Design review of the part built by this model. Coordinates are the model's own, in mm. A direction names the side the tool comes from. Coordinates: 2 decimals unless noted, no trailing zeros. Loops run counter-clockwise (first coordinate to the right, second up) from the corner with the lowest first, then second, coordinate; pieces in that order, holes last.
Q1. Draft analysis for pull direction Y (two halves, no side actions). For faces 1 (the face through (-9.425, -6.386, 1.479)), 2 (the face through (27.5, 9, 1)), 3 (the face through (11.33, -5.69, 1.48)), 4 (the face through (-21.797, -18.986, 1.521)), state which applies: released by +Y, released by -Y, zero draft, split by the parting line, or undercut.
Q2. Wall thickness on probe 1 along X at (y, z) = (10, 1.4); probe 2 along X at (y, z) = (-5, 1.4); probe 3 along Y at (x, z) = (20, 0.3): over which ranges is each line inside the solid? List them lowest first.
Q3. Add section D-D on y = -22. Give the boundary of the cut face in (x, z), and give its area (3 significant figures).
Q4. Add section B-B on z = 2.05. Give the boundary of the cut face in (x, y).
Q5. For P1, Ø1, axis at y = 26, z = 1.5, coming from the -X side; P2, Ø1, axis at y = 26.5, z = 1, coming from the +X side; P3, Ø1.5, axis at x = -18.5, z = 1.5, coming from the +Y side, all flat-tipped, find the tip position at first contact; note any pin that passes through.
Q6. Add section C-C on x = -20. Give the boundary of the cut face in (y, z), and give its area (3 significant figures).
Q7. Machinability: for faces 5 (the face through (-21.01, 8.89, 1.52)), 6 (the face through (-18, 25, 1)), 7 (the face through (18, 25, 1)), which of the approach directions +Z, -Z, +X, -X, +Y, -Y give a long, thin tool a straight path to every point of the face, cutting with its end or side? Answer none if there is none.
Q8. Add section A-A on y = 10. Give the boundary of the cut face in (x, z).
Autodesk Inventor part; units mm, degrees
ref_plane "YZ Plane" through (0, 0, 0) normal (1, 0, 0) x (0, 1, 0)
ref_plane "XZ Plane" through (0, 0, 0) normal (0, 1, 0) x (-1, 0, 0)
ref_plane "XY Plane" through (0, 0, 0) normal (0, 0, 1) x (1, 0, 0)
sketch "Boceto1" plane through (0, 0, 0) normal (0, 0, 1) x (1, 0, 0)
  line L0 (-27.5, -25) -> (27.5, -25)
  line L1 (27.5, -25) -> (27.5, 25)
  line L2 (27.5, 25) -> (-27.5, 25)
  line L3 (-27.5, 25) -> (-27.5, -25)
  line L4 (-27.5, -25) -> (27.5, 25) construction
  line L5 (27.5, -25) -> (-27.5, 25) construction
  point P0 (0, 0)
  dimension "d0" = 55
  dimension "d1" = 50
extrude "Extrusión1" add sketch "Boceto1" along normal blind 3
sketch "Boceto2" plane through (0, 0, 3) normal (0, 0, 1) x (1, 0, 0)
  line L0 (-10, 22) -> (10, 22)
  line L1 (10, 22) -> (10, 28)
  line L2 (10, 28) -> (-10, 28)
  line L3 (-10, 28) -> (-10, 22)
  line L4 (27.5, 25) -> (-27.5, 25) construction
  line L5 (-10, 22) -> (10, 28) construction
  line L6 (10, 22) -> (-10, 28) construction
  point P0 (0, 0)
  point P1 (0, 25)
  dimension "d4" = 20
  dimension "d5" = 6
extrude "Extrusión2" add sketch "Boceto2" against normal up to surface (3 mm away)
fillet "Empalme1" radius 1 4 edges at (-27.5, 25, 1.5) (27.5, 25, 1.5) (10, 28, 1.5) (-10, 28, 1.5)
sketch "Boceto3" plane through (0, 0, 0) normal (0, 0, -1) x (-1, 0, 0)
  circle A0 centre (20, 10) radius 1.6 construction
  circle A1 centre (10, 10) radius 1.6 construction
  circle A2 centre (-10, 10) radius 1.6 construction
  circle A3 centre (-20, 10) radius 1.6 construction
  point P0 (0, 0)
hole "Agujero1" at (20, 10, 0) at (10, 10, 0) at (-10, 10, 0) at (-20, 10, 0) direction (0, 0, 1) diameter 3 end through all
sketch "Boceto4" plane through (0, 0, 3) normal (0, 0, 1) x (1, 0, 0)
  line L0 (-27.5, -25) -> (27.5, -25) construction
  line L1 (-27.5, 24) -> (-27.5, -25) construction
  line L2 (0, -35.6) -> (0, 38.6) construction
  line L3 (-10, 25) -> (-26.5, 25) construction
  point P0 (0, 0)
  point P1 (-10, -5)
  point P2 (-26.5, -25)
  point P3 (26.5, -25)
  point P4 (-27.5, -24)
  dimension "d18" = 10
  dimension "d26" = 30
hole "Agujero2" at (-10, -5, 3) direction (0, 0, -1) diameter 3 end through all
mirror "Simetría1" about plane through (0, 0, 0) normal (1, 0, 0) of "Agujero2"
fillet "Empalme2" radius 20 2 edges at (-27.5, -25, 1.5) (27.5, -25, 1.5)
properties part number "PlacaBaseGarraSTD"
Entries:
1. face 1: undercut
1. face 2: zero draft
1. face 3: undercut
1. face 4: released by -Y
2. probe 1: x = -27.5 to -21.5, -18.5 to -11.5, -8.5 to 8.5, 11.5 to 18.5, 21.5 to 27.5
2. probe 2: x = -27.5 to -11.5, -8.5 to 8.5, 11.5 to 27.5
2. probe 3: y = -20.61 to 8.5, 11.5 to 25
3. outline: (-18.04, 0) - (18.04, 0) - (18.04, 3) - (-18.04, 3) - close
3. area: 108 mm2
4. outline: (-27.5, -5) arc R20 ccw to (-7.5, -25) - (7.5, -25) arc R20 ccw to (27.5, -5) - (27.5, 24) arc R1 ccw to (26.5, 25) - (10, 25) - (10, 27) arc R1 ccw to (9, 28) - (-9, 28) arc R1 ccw to (-10, 27) - (-10, 25) - (-26.5, 25) arc R1 ccw to (-27.5, 24) - close; hole circle Ø3 at (-20, 10); hole circle Ø3 at (-10, -5); hole circle Ø3 at (-10, 10); hole circle Ø3 at (10, -5); hole circle Ø3 at (10, 10); hole circle Ø3 at (20, 10)
5. P1: stops at x = -10
5. P2: stops at x = 10
5. P3: stops at y = 25
6. outline: (-20.61, 0) - (8.5, 0) - (8.5, 3) - (-20.61, 3) - close; (11.5, 0) - (25, 0) - (25, 3) - (11.5, 3) - close
6. area: 128 mm2
7. face 5: +Z, -Z
7. face 6: +Z, -Z, -X, +Y
7. face 7: +Z, -Z, +X, +Y
8. outline: (-27.5, 0) - (-21.5, 0) - (-21.5, 3) - (-27.5, 3) - close; (-18.5, 0) - (-11.5, 0) - (-11.5, 3) - (-18.5, 3) - close; (-8.5, 0) - (8.5, 0) - (8.5, 3) - (-8.5, 3) - close; (11.5, 0) - (18.5, 0) - (18.5, 3) - (11.5, 3) - close; (21.5, 0) - (27.5, 0) - (27.5, 3) - (21.5, 3) - close
